For this review, take the finished solid that the model builds, in its own axes (mm). A direction names the side the tool comes from. Round coordinates to 2 decimals unless told otherwise and drop trailing zeros. Loops run counter-clockwise (first coordinate to the right, second up) from the corner with the lowest first, then second, coordinate; pieces in that order, holes last. Notation, with made-up numbers: M 15,-31.75 L 52,-31.75 A4 cw 52,-27.75 Z; hole C -13,75.5 d1. An arc over 180 degrees is marked long. One line per question, with ' | ' between items. Start each with the question number.
1) For faces 5 (the face through (5, -2, 4)), 6 (the face through (-1.73, -7.81, -4.37)), 7 (the face through (0, 10, 4.75)), list the 3-axis set-ups (+Z, -Z, +X, -X, +Y, -Y) from which the entire face can be reached by the end or side of a thin tool; tool diameter is ignored.
2) We need section A-A (z = 0). Give the boundary of the cut face in (x, y).
3) For pin 1 Ø8 at (x, y) = (-3.5, 100) entering from -Z; pin 2 Ø12 at (x, z) = (2, 0.5) entering from +Y; pin 3 Ø12 at (x, y) = (13, 120) entering from +Z; pin 4 Ø17.5 at (x, y) = (-7.5, -1.5) entering from -Z, all flat-tipped, find the tip position at first contact; note any pin that passes through.
4) We need section C-C (y = 0). Give the boundary of the cut face in (x, z).
5) For probe 1 along X at (y, z) = (76, 0); probe 2 along Y at (x, z) = (0, -4.2); probe 3 along Z at (x, y) = (-15, 65.5), list the stretches that pass through material, from the lowest coordinate up. Write a range as from..to.
6) We need section D-D (y = 153). Give the boundary of the cut face in (x, z), and give its area (3 significant figures).
7) Mouldability with a two-part tool opening along X and no side actions: class faces 1 (the face through (0, 46, 0)), 2 (the face through (0.24, 14.5, -6.18)), 3 (the face through (-16.855, 102.118, -2.213)), 4 (the face through (-5.37, 106.84, -1.19)) as pulls with the +X half, pulls with the -X half, needs draft (parallel to the pull), parting line crosses it, or undercut.
```python
from build123d import *

# Parameters (mm, degrees)
CUT_EXTRUDE1_DEPTH = 25
CUT_EXTRUDE2_START = -4
SKETCH4_R          = 8
CUT_EXTRUDE2_DEPTH = 4
CUT_EXTRUDE3_START = 8
SKETCH4_2_R        = 8
CUT_EXTRUDE3_DEPTH = 4
SKETCH5_R          = 5.5
CUT_EXTRUDE4_DEPTH = 120


with BuildPart() as part:
    # Sketch1 → Revolve1 (revolve)
    with BuildSketch(Plane.XY, mode=Mode.PRIVATE) as revolve1_sk:
        with BuildLine():
            Line((0, 166), (-17, 166))
            Line((-17, 166), (-17, 40))
            Line((-17, 40), (-19.6, 40))
            Line((-19.6, 40), (-19.6, 18))
            Line((-19.6, 18), (-11.23029167, -4.228539819))
            ThreePointArc((-11.23029167, -4.228539819), (-6.828525543, -9.867686604), (0, -12))
            Line((0, -12), (0, 166))
        make_face()
    revolve(revolve1_sk.sketch.rotate(Axis((0, 166, 0), (0, -1, 0)), 270), axis=Axis((0, 166, 0), (0, -1, 0)))

    # Sketch2 → Cut-Extrude1 (cut, symmetric)
    with BuildSketch(Plane(origin=(0, 0, 0), x_dir=(0, 0, -1), z_dir=(1, 0, 0))):
        with BuildLine():
            Line((-4.75, -11.548161577), (-4.75, 11))
            ThreePointArc((-4.75, 11), (-6.214466094, 14.535533906), (-9.75, 16))
            Line((-9.75, 16), (-25.870257209, 16))
            Line((-25.870257209, 16), (-25.870257209, -11.548161577))
            Line((-25.870257209, -11.548161577), (-4.75, -11.548161577))
        make_face()
        with BuildLine():
            Line((25.870257209, 16), (25.870257209, -11.548161577))
            Line((25.870257209, -11.548161577), (4.75, -11.548161577))
            Line((4.75, -11.548161577), (4.75, 11))
            ThreePointArc((4.75, 11), (6.214466094, 14.535533906), (9.75, 16))
            Line((9.75, 16), (25.870257209, 16))
        make_face()
    extrude(amount=CUT_EXTRUDE1_DEPTH, both=True, mode=Mode.SUBTRACT)

    # Sketch3 → Cut-Revolve1 (revolve, cut)
    with BuildSketch(Plane.XY):
        with BuildLine():
            Line((0, -6.5), (0, 6.5))
            ThreePointArc((0, 6.5), (-6.5, 0), (0, -6.5))
        make_face()
    revolve(axis=Axis((0, -12, 0), (0, 1, 0)), mode=Mode.SUBTRACT)

    # Sketch4 → Cut-Extrude2 (cut)
    with BuildSketch(Plane.XY.offset(CUT_EXTRUDE2_START)):
        Circle(SKETCH4_R)
    extrude(amount=-CUT_EXTRUDE2_DEPTH, mode=Mode.SUBTRACT)

    # Sketch4_2 → Cut-Extrude3 (cut)
    with BuildSketch(Plane.XY.offset(CUT_EXTRUDE3_START)):
        Circle(SKETCH4_2_R)
    extrude(amount=-CUT_EXTRUDE3_DEPTH, mode=Mode.SUBTRACT)

    # Sketch5 → Cut-Extrude4 (cut)
    with BuildSketch(Plane(origin=(0, 166, 0), x_dir=(1, 0, 0), z_dir=(0, 1, 0))):
        with Locations(Location((0, 0, 0), (0, 0, 270))):
            Circle(SKETCH5_R)
    extrude(amount=-CUT_EXTRUDE4_DEPTH, mode=Mode.SUBTRACT)


solid = part.part
```
Answers below:
1) face 5: +Z | face 6: -Z | face 7: +Z, +X, -X, -Y
2) outline: M -19.6,18 L -11.23,-4.23 A12 ccw 11.23,-4.23 L 19.6,18 L 19.6,40 L 17,40 L 17,166 L 5.5,166 L 5.5,46 L -5.5,46 L -5.5,166 L -17,166 L -17,40 L -19.6,40 Z; hole C 0,0 d13
3) pin 1: z = -17 | pin 2: y = 166 | pin 3: z = 15.49 | pin 4: z = -4.75
4) outline: M -11.91,-4.75 L -8,-4.75 L -8,-4 L -5.12,-4 A6.5 cw -5.12,4 L -8,4 L -8,4.75 L -11.91,4.75 A12.82 ccw Z; M 5.12,-4 L 8,-4 L 8,-4.75 L 11.91,-4.75 A12.82 ccw 11.91,4.75 L 8,4.75 L 8,4 L 5.12,4 A6.5 cw Z
5) probe 1: -17..-5.5, 5.5..17 | probe 2: -11.24..-8, 8..46 | probe 3: -8..8
6) outline: C 0,0 d34; hole C 0,0 d11 | area: 813 mm^2
7) face 1: undercut | face 2: needs draft | face 3: parting line crosses it | face 4: undercut
